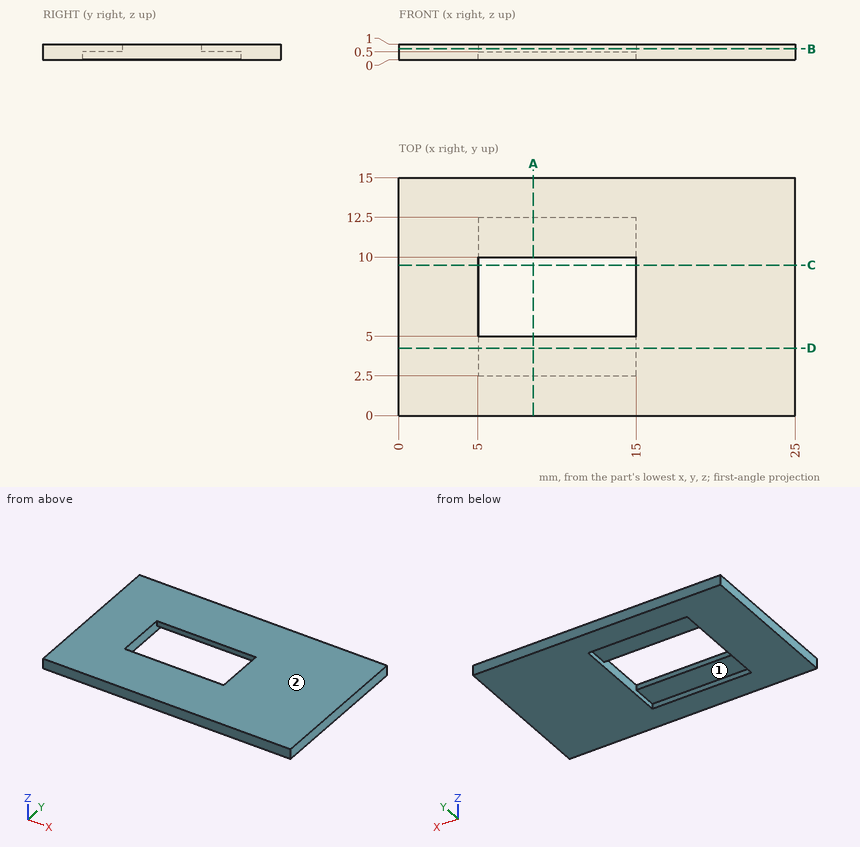
Study the drawing (mm; zero at the part's minimum x, y, z) and answer. Round coordinates to 2 decimals unless told otherwise and drop trailing zeros. Write each loop counter-clockwise with the first axis right and the second up, starting at its lowest first coordinate (ties: lowest second). Pieces come first, ordered by that corner, then holes.
1) A cutting plane is placed at D-D (y = 4.25). Give the vertices of the cut face in (x, z), plus the area to 3 significant figures.
2) A cutting plane is placed at A-A (x = 8.5). Give the vertices of the cut face in (y, z), plus the area to 3 significant figures.
3) A cutting plane is placed at B-B (z = 0.7). Give the vertices of the cut face in (x, y), plus the area to 3 significant figures.
4) A cutting plane is placed at C-C (y = 9.5). Give the vertices of the cut face in (x, z), plus the area to 3 significant figures.
5) Given pin 1 Ø1.2 at (x, y) = (11.5, 10.5) entering from -Z, flat-ended and moving along its own axis, determine where the tip first touches the part or whether it passes through.
6) Straight lines are drawn through the part: line 1 (Y direction, x = 14, z = 0.3); line 2 (X direction, y = 5.75, z = 0.95); line 3 (Z direction, x = 12, y = 12.25). For each, find the intervals that lie inside material, in ascending order.
7) The mould has two halves that part along X. Classify the marked faces 1 and 2: pulls with the +X half, pulls with the -X half, needs draft (parallel to the pull), parting line crosses it, or undercut.
Completed:
1. outline: (0, 0) - (5, 0) - (5, 0.5) - (15, 0.5) - (15, 0) - (25, 0) - (25, 1) - (0, 1) - close
1. area: 20.0 mm2
2. outline: (0, 0) - (2.5, 0) - (2.5, 0.5) - (5, 0.5) - (5, 1) - (0, 1) - close; (10, 0.5) - (12.5, 0.5) - (12.5, 0) - (15, 0) - (15, 1) - (10, 1) - close
2. area: 7.50 mm2
3. outline: (0, 0) - (25, 0) - (25, 15) - (0, 15) - close; hole (5, 5) - (15, 5) - (15, 10) - (5, 10) - close
3. area: 325 mm2
4. outline: (0, 0) - (5, 0) - (5, 1) - (0, 1) - close; (15, 0) - (25, 0) - (25, 1) - (15, 1) - close
4. area: 15.0 mm2
5. pin 1: stops at z = 0.5
6. line 1: y = 0 to 2.5, 12.5 to 15
6. line 2: x = 0 to 5, 15 to 25
6. line 3: z = 0.5 to 1
7. face 1: undercut
7. face 2: needs draft
